```python
from build123d import *

# Parameters (mm, degrees)
SKETCH1_W           = 17.6609375
SKETCH1_H           = 12.1046875
BOSS_EXTRUDE1_DEPTH = 7.9375
SKETCH2_W           = 11.43
SKETCH2_H           = 4.7625
CUT_EXTRUDE1_DEPTH  = 25.4
SKETCH3_R           = 2.1828125
CUT_EXTRUDE2_DEPTH  = 25.4


with BuildPart() as part:
    # Sketch1 → Boss-Extrude1 (new body)
    with BuildSketch(Plane(origin=(0, 0, 0), x_dir=(1, 0, 0), z_dir=(0, 1, 0))):
        with Locations((8.83046875, 6.05234375)):
            Rectangle(SKETCH1_W, SKETCH1_H)
    extrude(amount=BOSS_EXTRUDE1_DEPTH)

    # Sketch2 → Cut-Extrude1 (cut)
    with BuildSketch(Plane.XY):
        with Locations((5.715, 5.55625)):
            Rectangle(SKETCH2_W, SKETCH2_H)
    extrude(amount=-CUT_EXTRUDE1_DEPTH, mode=Mode.SUBTRACT)

    # Sketch3 → Cut-Extrude2 (cut)
    with BuildSketch(Plane(origin=(0, 3.175, 0), x_dir=(1, 0, 0), z_dir=(0, 1, 0))):
        with Locations(Location((4.1671875, 6.35, 0), (0, 0, 270))):
            Circle(SKETCH3_R)
    extrude(amount=-CUT_EXTRUDE2_DEPTH, mode=Mode.SUBTRACT)


solid = part.part
```
Source: CAD feature listing. Evaluate the final solid. Frame: model axes, mm. A direction names the side the tool comes from. Round coordinates to 2 decimals unless told otherwise and drop trailing zeros. Loops run counter-clockwise (first coordinate to the right, second up) from the corner with the lowest first, then second, coordinate; pieces in that order, holes last.
1. Mould query, pull axis Z, two halves, no side actions, for faces 1 (the flat face through (11, 3, -12.105)), 2 (the cylindrical face through (4.26, 1.61, -8.53)), 3 (the flat face through (7, 3.175, -6)). Classes: released by +Z, released by -Z, zero draft, split by the parting line, or undercut.
2. Section query D-D on y = 6.5. Output: boundary loops of the cut face in (x, z).
3. Ray query, L1, parallel to X at y = 1, z = -6.35; L2, parallel to Y at x = 6.25, z = -0.25 (3 decimals); L3, parallel to X at y = 5, z = -2.25. Return the intervals inside material, ascending.
4. Section query B-B on z = -8.75. Output: boundary loops of the cut face in (x, y) (1 decimal), and give its area (3 significant figures).
5. Section query C-C on x = 8.5. Output: boundary loops of the cut face in (y, z) (3 decimals).
6. Access query for faces 4 (the flat face through (11.43, 6, -6)), 5 (the flat face through (11, 3, 0)). Directions: +Z, -Z, +X, -X, +Y, -Y. A direction counts if a zero-diameter tool reaches every point of the face in a straight line with its end or side. Return the directions, or none.
Answers below:
1. face 1: released by -Z
1. face 2: undercut
1. face 3: zero draft
2. outline: (11.43, -12.1) - (17.66, -12.1) - (17.66, 0) - (11.43, 0) - close
3. L1: x = 0 to 1.98, 6.35 to 17.66
3. L2: y = 0 to 3.175
3. L3: x = 11.43 to 17.66
4. outline: (0, 0) - (17.7, 0) - (17.7, 7.9) - (11.4, 7.9) - (11.4, 3.2) - (0, 3.2) - close
4. area: 85.7 mm2
5. outline: (0, -12.105) - (3.175, -12.105) - (3.175, 0) - (0, 0) - close
6. face 4: +Z, -Z, -X, +Y
6. face 5: +Z, +X, -X, +Y, -Y
